The drawing under review shows one solid part. Ordinate dimensions are in mm from its lowest x, y, z. Round coordinates to 2 decimals unless told otherwise and drop trailing zeros. Order: outer loops, then holes, each group sorted by start corner. A loop starts at its lowest first (then second) coordinate and runs counter-clockwise, first axis right, second up. Notation, with made-up numbers: (-28.5, -16.5) -> (-4.5, -16.5) arc R10 ccw to (-4.5, -0.5) -> close; hole circle Ø4 at (72.25, 65). An arc over 180 degrees is marked (long way). Use a Markdown table: item, result. Add a question column.
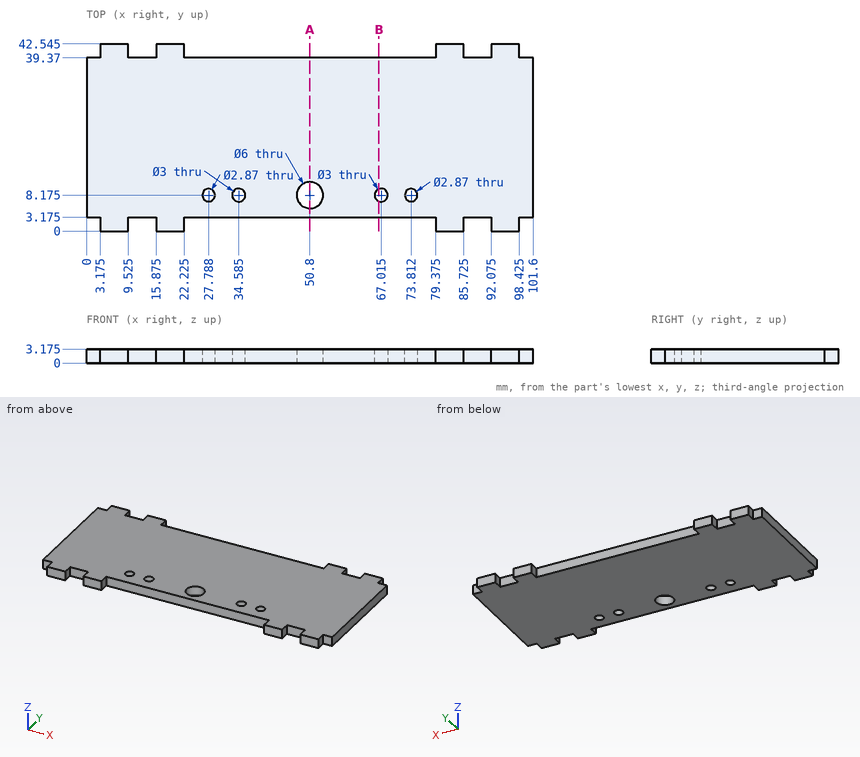
Q1. Add section B-B, the plane x = 66.5. Give the boundary of the cut face in (y, z) (1 decimal), then the cut area to 3 significant figures.
Q2. Add section A-A, the plane x = 50.8. Give the boundary of the cut face in (y, z) (1 decimal).
Q3. For pin 1 (1 mm diameter, centred on x = 25.5, z = 2, fed in from -Y) (1 decimal); pin 2 (2.5 mm diameter, centred on x = 73.81, y = 8.18, fed in from -Z); pin 3 (4 mm diameter, centred on x = 34.585, y = 8.175, fed in from +Z) (1 decimal); pin 4 (1 mm diameter, centred on y = 41.5, z = 1, fed in from -X) (1 decimal), all flat-tipped, find the tip position at first contact; note any pin that passes through.
Q4. To check wall thickness, follow line 1 along X through (y, z) = (40.5, 2.85) (1 decimal); line 2 along Y through (x, z) = (50.8, 1.25) (1 decimal); line 3 along Y through (x, z) = (67, 1.9) (1 decimal). State the ranges of each line that lie inside material, in increasing order.
Return value:
| question | item | result |
|---|---|---|
| 1 | outline | (3.2, 0) -> (6.8, 0) -> (6.8, 3.2) -> (3.2, 3.2) -> close; (9.6, 0) -> (39.4, 0) -> (39.4, 3.2) -> (9.6, 3.2) -> close |
| 1 | area | 106 mm² |
| 2 | outline | (3.2, 0) -> (5.2, 0) -> (5.2, 3.2) -> (3.2, 3.2) -> close; (11.2, 0) -> (39.4, 0) -> (39.4, 3.2) -> (11.2, 3.2) -> close |
| 3 | pin 1 | y = 3.2 |
| 3 | pin 2 | through |
| 3 | pin 3 | z = 3.2 |
| 3 | pin 4 | x = 3.2 |
| 4 | line 1 | 3.2 to 9.5, 15.9 to 22.2, 79.4 to 85.7, 92.1 to 98.4 |
| 4 | line 2 | 3.2 to 5.2, 11.2 to 39.4 |
| 4 | line 3 | 3.2 to 6.7, 9.7 to 39.4 |
